Read the model definition and answer for the solid it produces. Units are mm, in the model's axes. A direction names the side the tool comes from. Give positions to 0.01 mm unless a question says otherwise; leave off trailing zeros. Loops run counter-clockwise (first coordinate to the right, second up) from the corner with the lowest first, then second, coordinate; pieces in that order, holes last. Notation, with made-up numbers: (85.25, 53.25) -> (136.25, 53.25) arc R32 cw to (136.25, 87.25) -> close; hole circle Ø6 at (56, 57). An arc over 180 degrees is marked (long way). Write each question's results on one line, items separated by ' | '. Start each with the question number.
Item 1: Find the intervals of material crossed by line 1 (Y direction, x = 0, z = 0.4); line 2 (Z direction, x = 0.5, y = -2); line 3 (Y direction, x = 3.5, z = 2.25), in increasing order.
Item 2: Section C-C on z = 2.75 is taken. Write down the section's boundary in (x, y).
Item 3: Section A-A on x = 0 is taken. Write down the section's boundary in (y, z), and give its area (3 significant figures).
Item 4: Each of these flat-tipped pins is pushed along its axis until it touches: P1, Ø1.5, axis at y = 3.5, z = 9, coming from the -X side; P2, Ø3, axis at x = 0.5, z = 10, coming from the -Y side. Where does it stop, or does it pass through?
Item 5: Section B-B on y = 0 is taken. Write down the section's boundary in (x, z).
Item 6: Determine the mould class of faces 1 (the cylindrical face through (-1.4, 0.06, 0.51)), 2 (the flat face through (4, 4.4, 5)), 3 (the flat face through (0, 4, 8)) for opening direction X: +X half, -X half, draft (parallel to the pull), parting line (faces both ways), or undercut.
Item 7: Section D-D on x = 2 is taken. Write down the section's boundary in (y, z), and give its area (3 significant figures).
Item 8: Which of the six approach directions +Z, -Z, +X, -X, +Y, -Y give full straight-line access (tool end or side, diameter ignored) to faces 4 (the flat face through (-0.9, -1.4, 1)), 5 (the flat face through (-0.1, 4.5, 16))?
```python
from build123d import *

# Parameters (mm, degrees)
SKETCH_W     = 8
SKETCH_H     = 10
PAD_DEPTH    = 1
SKETCH001_W  = 8
SKETCH001_H  = 1
PAD001_DEPTH = 15
SKETCH002_R  = 1.4
POCKET_DEPTH = 1


with BuildPart() as part:
    # Sketch → Pad (new body)
    with BuildSketch(Plane.XY):
        Rectangle(SKETCH_W, SKETCH_H)
    extrude(amount=PAD_DEPTH)

    # Sketch001 (on Face6 of Pad) → Pad001 (join)
    with BuildSketch(Plane.XY.offset(1)):
        with Locations((0, 4.5)):
            Rectangle(SKETCH001_W, SKETCH001_H)
    extrude(amount=PAD001_DEPTH)

    # Sketch002 (on Face5 of Pad001) → Pocket (cut)
    with BuildSketch(Plane.XY.offset(1)):
        Circle(SKETCH002_R)
    extrude(amount=-POCKET_DEPTH, mode=Mode.SUBTRACT)


solid = part.part
```
Findings:
1) line 1: -5 to -1.4, 1.4 to 5 | line 2: 0 to 1 | line 3: 4 to 5
2) outline: (-4, 4) -> (4, 4) -> (4, 5) -> (-4, 5) -> close
3) outline: (-5, 0) -> (-1.4, 0) -> (-1.4, 1) -> (-5, 1) -> close; (1.4, 0) -> (5, 0) -> (5, 16) -> (4, 16) -> (4, 1) -> (1.4, 1) -> close | area: 22.2 mm2
4) P1: x = -4 | P2: y = 4
5) outline: (-4, 0) -> (-1.4, 0) -> (-1.4, 1) -> (-4, 1) -> close; (1.4, 0) -> (4, 0) -> (4, 1) -> (1.4, 1) -> close
6) face 1: undercut | face 2: +X half | face 3: draft
7) outline: (-5, 0) -> (5, 0) -> (5, 16) -> (4, 16) -> (4, 1) -> (-5, 1) -> close | area: 25.0 mm2
8) face 4: +Z, +X, -X, -Y | face 5: +Z, +X, -X, +Y, -Y
